from build123d import *

# Parameters (mm, degrees)
EXTRUIR1_DEPTH         = 9.9
CROQUIS2_R             = 1
CORTAR_EXTRUIR1_DEPTH  = 15.9
CORTAR_EXTRUIR2_DEPTH  = 4
CROQUIS4_W             = 35
CROQUIS4_H             = 2.727458855
CORTAR_EXTRUIR3_DEPTH  = 24
CROQUIS5_W             = 35
CROQUIS5_H             = 3.2
CORTAR_EXTRUIR4_DEPTH  = 8.5
CROQUIS6_W             = 39
CROQUIS6_H             = 14.452712812
CORTAR_EXTRUIR5_DEPTH  = 3
EXTRUIR2_DEPTH         = 0.2
CROQUIS8_W             = 49.57319474
CROQUIS8_H             = 11.75
CORTAR_EXTRUIR6_DEPTH  = 0.5
CROQUIS9_W             = 2.460261438
CROQUIS9_H             = 4
CORTAR_EXTRUIR7_DEPTH  = 1
CHAFL_N1_SIZE          = 0.5
CHAFL_N2_SIZE          = 0.5
CROQUIS10_W            = 32.2
CROQUIS10_H            = 2.9
EXTRUIR3_DEPTH         = 5.5
CROQUIS11_W            = 10.5
CROQUIS11_H            = 1.5
CORTAR_EXTRUIR8_DEPTH  = 2.5
CROQUIS12_W            = 16
CROQUIS12_H            = 2
CORTAR_EXTRUIR9_DEPTH  = 57.5
CROQUIS13_W            = 35
CROQUIS13_H            = 3.2
CORTAR_EXTRUIR10_DEPTH = 0.7
CROQUIS15_W            = 5.5
CROQUIS15_H            = 7.9
EXTRUIR4_DEPTH         = 0.5
CHAFL_N3_SIZE          = 0.5
CROQUIS16_W            = 3
CROQUIS16_H            = 6.5
CORTAR_EXTRUIR11_DEPTH = 1
CHAFL_N4_SIZE          = 0.5
CORTAR_EXTRUIR12_DEPTH = 1
CHAFL_N5_SIZE          = 0.5
CHAFL_N6_SIZE          = 0.5
CROQUIS18_W            = 0.4398817
CROQUIS18_H            = 4
CORTAR_EXTRUIR13_DEPTH = 22
CROQUIS19_W            = 10.696044144
CROQUIS19_H            = 2.8
CORTAR_EXTRUIR14_DEPTH = 0.2
CROQUIS20_W            = 2
CROQUIS20_H            = 4
CORTAR_EXTRUIR15_DEPTH = 0.2
CROQUIS21_W            = 42.865199157
CROQUIS21_H            = 3.067417921
CORTAR_EXTRUIR16_DEPTH = 58


with BuildPart() as part:
    # Croquis1 → Extruir1 (new body)
    with BuildSketch(Plane(origin=(0, 0, 0), x_dir=(1, 0, 0), z_dir=(0, 1, 0))):
        Polygon((23.5, 0), (-23.5, 0), (-23.5, -35), (-20.6, -35), (-20.6, -6.7), (20.6, -6.7), (20.6, -35), (23.5, -35), align=None)
    extrude(amount=EXTRUIR1_DEPTH)

    # Croquis2 → Cortar-Extruir1 (cut)
    with BuildSketch(Plane(origin=(0, 9.9, 0), x_dir=(-1, 0, 0), z_dir=(0, 1, 0))):
        with Locations((-20.08, 3)):
            Circle(CROQUIS2_R)
        with Locations((20.08, 3)):
            Circle(CROQUIS2_R)
    extrude(amount=-CORTAR_EXTRUIR1_DEPTH, mode=Mode.SUBTRACT)

    # Croquis3 → Cortar-Extruir2 (cut)
    with BuildSketch(Plane(origin=(0, 9.9, 0), x_dir=(-1, 0, 0), z_dir=(0, 1, 0))):
        Polygon((-20.08, 5.5), (-22.245063509, 4.25), (-22.245063509, 1.75), (-20.08, 0.5), (-17.914936491, 1.75), (-17.914936491, 4.25), align=None)
        Polygon((20.08, 5.5), (17.914936491, 4.25), (17.914936491, 1.75), (20.08, 0.5), (22.245063509, 1.75), (22.245063509, 4.25), align=None)
    extrude(amount=-CORTAR_EXTRUIR2_DEPTH, mode=Mode.SUBTRACT)

    # Croquis4 → Cortar-Extruir3 (cut)
    with BuildSketch(Plane(origin=(0, 9.9, 0), x_dir=(-1, 0, 0), z_dir=(0, 1, 0))):
        with Locations((0, 0.136270572)):
            Rectangle(CROQUIS4_W, CROQUIS4_H)
    extrude(amount=-CORTAR_EXTRUIR3_DEPTH, mode=Mode.SUBTRACT)

    # Croquis5 → Cortar-Extruir4 (cut)
    with BuildSketch(Plane(origin=(0, 9.9, 0), x_dir=(-1, 0, 0), z_dir=(0, 1, 0))):
        with Locations((0, 3.1)):
            Rectangle(CROQUIS5_W, CROQUIS5_H)
    extrude(amount=-CORTAR_EXTRUIR4_DEPTH, mode=Mode.SUBTRACT)

    # Croquis6 → Cortar-Extruir5 (cut)
    with BuildSketch(Plane(origin=(0, 9.9, 0), x_dir=(-1, 0, 0), z_dir=(0, 1, 0))):
        with Locations((0, 5.388219545)):
            Rectangle(CROQUIS6_W, CROQUIS6_H)
    extrude(amount=-CORTAR_EXTRUIR5_DEPTH, mode=Mode.SUBTRACT)

    # Croquis7 → Extruir2 (add)
    with BuildSketch(Plane(origin=(0, 3.9, 0), x_dir=(-1, 0, 0), z_dir=(0, 1, 0))):
        with BuildLine():
            Line((-20.6, 35), (-19.5, 35))
            Line((-19.5, 35), (-19.080611376, 14.617712891))
            ThreePointArc((-19.080611376, 14.617712891), (-17.880640918, 11.842628092), (-15.081457862, 10.7))
            Line((-15.081457862, 10.7), (15.081457862, 10.7))
            ThreePointArc((15.081457862, 10.7), (17.880640918, 11.842628092), (19.080611376, 14.617712891))
            Line((19.080611376, 14.617712891), (19.5, 35))
            Line((19.5, 35), (20.6, 35))
            Line((20.6, 35), (20.6, 6.7))
            Line((20.6, 6.7), (-20.6, 6.7))
            Line((-20.6, 6.7), (-20.6, 35))
        make_face()
    extrude(amount=-EXTRUIR2_DEPTH)

    # Croquis8 → Cortar-Extruir6 (cut)
    with BuildSketch(Plane(origin=(0, 9.9, 0), x_dir=(-1, 0, 0), z_dir=(0, 1, 0))):
        with Locations((0.155531932, 7.625)):
            Rectangle(CROQUIS8_W, CROQUIS8_H)
    extrude(amount=-CORTAR_EXTRUIR6_DEPTH, mode=Mode.SUBTRACT)

    # Croquis9 → Cortar-Extruir7 (cut)
    with BuildSketch(Plane(origin=(0, 9.9, 0), x_dir=(-1, 0, 0), z_dir=(0, 1, 0))):
        with Locations((23.330130719, 19)):
            Rectangle(CROQUIS9_W, CROQUIS9_H)
        with Locations((-23.330130719, 19)):
            Rectangle(CROQUIS9_W, CROQUIS9_H)
    extrude(amount=-CORTAR_EXTRUIR7_DEPTH, mode=Mode.SUBTRACT)

    # Chaflán1
    chafl_n1_edges = [part.edges().sort_by_distance(p)[0] for p in [
        (23.5, 9.9, 15.25),
        (23.5, 9.9, 28),
        (-23.5, 9.9, 28),
        (-23.5, 9.9, 15.25),
    ]]
    chamfer(chafl_n1_edges, length=CHAFL_N1_SIZE)

    # Chaflán2
    chafl_n2_edges = [part.edges().sort_by_distance(p)[0] for p in [
        (23.5, 9.9, 0.875),
        (-23.5, 9.9, 0.875),
    ]]
    chamfer(chafl_n2_edges, length=CHAFL_N2_SIZE)

    # Croquis10 → Extruir3 (add)
    with BuildSketch(Plane(origin=(0, 9.4, 0), x_dir=(-1, 0, 0), z_dir=(0, 1, 0))):
        with Locations((0, 6.15)):
            Rectangle(CROQUIS10_W, CROQUIS10_H)
    extrude(amount=-EXTRUIR3_DEPTH)

    # Croquis11 → Cortar-Extruir8 (cut)
    with BuildSketch(Plane(origin=(0, 9.4, 0), x_dir=(-1, 0, 0), z_dir=(0, 1, 0))):
        with Locations((-10.15, 6.15)):
            Rectangle(CROQUIS11_W, CROQUIS11_H)
        with Locations((10.15, 6.15)):
            Rectangle(CROQUIS11_W, CROQUIS11_H)
    extrude(amount=-CORTAR_EXTRUIR8_DEPTH, mode=Mode.SUBTRACT)

    # Croquis12 → Cortar-Extruir9 (cut)
    with BuildSketch(Plane.ZY.offset(23.5)):
        with Locations((15.5, 1)):
            Rectangle(CROQUIS12_W, CROQUIS12_H)
    extrude(amount=-CORTAR_EXTRUIR9_DEPTH, mode=Mode.SUBTRACT)

    # Croquis13 → Cortar-Extruir10 (cut)
    with BuildSketch(Plane.XZ):
        with Locations((0, 3.1)):
            Rectangle(CROQUIS13_W, CROQUIS13_H)
    extrude(amount=-CORTAR_EXTRUIR10_DEPTH, mode=Mode.SUBTRACT)

    # Croquis15 → Extruir4 (add)
    with BuildSketch(Plane.ZY.offset(23.5)):
        Polygon((4, 0), (4, 7.9), (23, 7.9), (23, 2), (7.5, 2), (7.5, 0), align=None)
        with Locations((32.25, 3.95)):
            Rectangle(CROQUIS15_W, CROQUIS15_H)
    extruir4 = extrude(amount=EXTRUIR4_DEPTH)

    # Chaflán3
    chafl_n3_edges = [part.edges().sort_by_distance(p)[0] for p in [
        (-23.75, 7.9, 29.5),
        (-23.75, 7.9, 23),
        (-23.75, 7.9, 4),
    ]]
    chamfer(chafl_n3_edges, length=CHAFL_N3_SIZE)

    # Croquis16 → Cortar-Extruir11 (cut)
    with BuildSketch(Plane.ZY.offset(23.5)):
        with Locations((28, 3.25)):
            Rectangle(CROQUIS16_W, CROQUIS16_H)
    cortar_extruir11 = extrude(amount=-CORTAR_EXTRUIR11_DEPTH, mode=Mode.SUBTRACT)

    # Simetría1: Extruir4, Cortar-Extruir11 across plane
    add(extruir4.mirror(Plane(origin=(0, 0, 0), x_dir=(0, 0, 1), z_dir=(1, 0, 0))))
    add(cortar_extruir11.mirror(Plane(origin=(0, 0, 0), x_dir=(0, 0, 1), z_dir=(1, 0, 0))), mode=Mode.SUBTRACT)

    # Chaflán4
    chafl_n4_edges = [part.edges().sort_by_distance(p)[0] for p in [
        (23.75, 7.9, 4),
        (23.75, 7.9, 23),
        (23.75, 7.9, 29.5),
    ]]
    chamfer(chafl_n4_edges, length=CHAFL_N4_SIZE)

    # Croquis17 → Cortar-Extruir12 (cut)
    with BuildSketch(Plane(origin=(-20.6, 0, 0), x_dir=(0, 0, -1), z_dir=(1, 0, 0))):
        Polygon((-35, 7.9), (-7.2, 7.9), (-7.2, 6.65), (-22.2, 6.65), (-22.2, 5.15), (-7.2, 5.15), (-7.2, 3.9), (-35, 3.9), align=None)
    cortar_extruir12 = extrude(amount=-CORTAR_EXTRUIR12_DEPTH, mode=Mode.SUBTRACT)

    # Chaflán5
    chafl_n5_edges = [part.edges().sort_by_distance(p)[0] for p in [
        (-20.6, 5.9, 22.2),
    ]]
    chamfer(chafl_n5_edges, length=CHAFL_N5_SIZE)

    # Simetría2: Cortar-Extruir12 across plane
    add(cortar_extruir12.mirror(Plane(origin=(0, 0, 0), x_dir=(0, 0, 1), z_dir=(1, 0, 0))), mode=Mode.SUBTRACT)

    # Chaflán6
    chafl_n6_edges = [part.edges().sort_by_distance(p)[0] for p in [
        (20.6, 5.9, 22.2),
    ]]
    chamfer(chafl_n6_edges, length=CHAFL_N6_SIZE)

    # Croquis18 → Cortar-Extruir13 (cut)
    with BuildSketch(Plane.XY.offset(35)):
        with Locations((-21.98005915, 5.9)):
            Rectangle(CROQUIS18_W, CROQUIS18_H)
        with Locations((21.98005915, 5.9)):
            Rectangle(CROQUIS18_W, CROQUIS18_H)
    extrude(amount=-CORTAR_EXTRUIR13_DEPTH, mode=Mode.SUBTRACT)

    # Croquis19 → Cortar-Extruir14 (cut)
    with BuildSketch(Plane(origin=(-21.6, 0, 0), x_dir=(0, 0, -1), z_dir=(1, 0, 0))):
        with Locations((-29.651977928, 5.9)):
            Rectangle(CROQUIS19_W, CROQUIS19_H)
    cortar_extruir14 = extrude(amount=-CORTAR_EXTRUIR14_DEPTH, mode=Mode.SUBTRACT)

    # Croquis20 → Cortar-Extruir15 (cut)
    with BuildSketch(Plane(origin=(-21.6, 0, 0), x_dir=(0, 0, -1), z_dir=(1, 0, 0))):
        with Locations((-34, 5.9)):
            Rectangle(CROQUIS20_W, CROQUIS20_H)
    cortar_extruir15 = extrude(amount=-CORTAR_EXTRUIR15_DEPTH, mode=Mode.SUBTRACT)

    # Simetría3: Cortar-Extruir14, Cortar-Extruir15 across plane
    add(cortar_extruir14.mirror(Plane(origin=(0, 0, 0), x_dir=(0, 0, 1), z_dir=(1, 0, 0))), mode=Mode.SUBTRACT)
    add(cortar_extruir15.mirror(Plane(origin=(0, 0, 0), x_dir=(0, 0, 1), z_dir=(1, 0, 0))), mode=Mode.SUBTRACT)

    # Croquis21 → Cortar-Extruir16 (cut)
    with BuildSketch(Plane(origin=(24, 0, 0), x_dir=(0, 0, -1), z_dir=(1, 0, 0))):
        with Locations((-17.067402922, -0.133708961)):
            Rectangle(CROQUIS21_W, CROQUIS21_H)
    extrude(amount=-CORTAR_EXTRUIR16_DEPTH, mode=Mode.SUBTRACT)


solid = part.part
Build history of the part. All positions in model axes, mm. A direction names the side the tool comes from. Round coordinates to 2 decimals unless told otherwise and drop trailing zeros. Write each loop counter-clockwise with the first axis right and the second up, starting at its lowest first coordinate (ties: lowest second). Pieces come first, ordered by that corner, then holes. Notation, with made-up numbers: M 66.5,65 L 93.5,65 A14 cw 93.5,80 Z; hole C 20,75.25 d11. An arc over 180 degrees is marked long. Use CSV: the item, a comma, the result in double quotes.
1. Saw through at B-B (x = 10). Give the cut face in (y, z), plus the area to 3 significant figures.
Reply:
outline,"M 1.4,4.7 L 9.4,4.7 L 9.4,5.4 L 6.9,5.4 L 6.9,6.9 L 9.4,6.9 L 9.4,7.6 L 3.9,7.6 L 3.9,10.7 L 3.7,10.7 L 3.7,6.7 L 1.4,6.7 Z"
area,"18.0 mm²"
2. Saw through at C-C (z = 9). Give the cut face in (x, y).
Reply:
outline,"M -24,2 L -20.6,2 L -20.6,3.7 L 20.6,3.7 L 20.6,2 L 24,2 L 24,7.9 L 23.5,7.9 L 23.5,9.4 L 20.6,9.4 L 20.6,7.9 L 21.6,7.9 L 21.6,6.65 L 20.6,6.65 L 20.6,5.15 L 21.6,5.15 L 21.6,3.9 L -21.6,3.9 L -21.6,5.15 L -20.6,5.15 L -20.6,6.65 L -21.6,6.65 L -21.6,7.9 L -20.6,7.9 L -20.6,9.4 L -23.5,9.4 L -23.5,7.9 L -24,7.9 Z"
3. Flat gauge pins, fed straight in: pin 1 (1.6 mm diameter, centred on x = -8, z = 6, fed in from +Y); pin 2 (3.5 mm diameter, centred on x = -18.5, z = 3.5, fed in from +Y). Where does each tip first touch, or does it go through?
Reply:
pin 1,"stops at y = 9.4"
pin 2,"stops at y = 6.9"
4. Tool access for faces 5 (the face through (0, 3.9, 10)), 6 (the face through (22.8, 9.4, 21)), 7 (the face through (21.178, 7.928, 1.134)), 8 (the face through (-20.6, 3, 21)): list every direction of +Z, -Z, +X, -X, +Y, -Y with a clear straight run to the whole face (end or side of a thin tool).
Reply:
face 5,"+Z"
face 6,"+X, +Y"
face 7,"+Y"
face 8,"+Z, -Y"
5. Saw through at A-A (z = 3). Give the cut face in (x, y), plus the area to 3 significant figures.
Reply:
outline,"M -23.5,1.4 L -21.08,1.4 L -21.08,5.9 L -22.25,5.9 L -22.25,9.4 L -23.5,9.4 Z; M -19.08,1.4 L -17.5,1.4 L -17.5,6.9 L -17.91,6.9 L -17.91,5.9 L -19.08,5.9 Z; M 17.5,1.4 L 19.08,1.4 L 19.08,5.9 L 17.91,5.9 L 17.91,6.9 L 17.5,6.9 Z; M 21.08,1.4 L 23.5,1.4 L 23.5,9.4 L 22.25,9.4 L 22.25,5.9 L 21.08,5.9 Z"
area,"45.6 mm²"
6. Wall check: probe 1 along X at (y, z) = (6.75, 2); probe 2 along Z at (x, y) = (20, 4); probe 3 along Y at (x, z) = (21, 19). Give the ranges that are in metal, low to high. Write a range as from..to.
Reply:
probe 1,"x = -23.5..-22.25, -17.91..-17.5, 17.5..17.91, 22.25..23.5"
probe 2,"z = 0..2, 4..6.7"
probe 3,"y = 2..3.9, 5.15..6.65, 7.9..9.9"
7. Two-plate mould, pull along Y, no slides. Class faces 1 (the face through (-22.2, 6, 24)), 2 (the face through (22.245, 8, 3)), 3 (the face through (0, 1.4, 5)), 4 (the face through (22, 9.9, 1)): +Y half, -Y half, draft (parallel to the pull), parting line (faces both ways), or undercut.
Reply:
face 1,"undercut"
face 2,"draft"
face 3,"-Y half"
face 4,"+Y half"
